from build123d import *

# Parameters (mm, degrees)
BOSS_EXTRUDE1_DEPTH          = 12.7
FILLET1_R                    = 19.05
F_10_0_1935_DIAMETER_HOLE1_D = 4.9149


with BuildPart() as part:
    # Sketch1 → Boss-Extrude1 (new body)
    with BuildSketch(Plane.ZY.offset(152.399999331)):
        Polygon((179.525, -30.525), (179.525, 10.75), (116.025, 179.025), (116.025, 191.725), (-116.025, 191.725), (-116.025, 179.025), (-179.525, 10.75), (-179.525, -30.525), align=None)
    extrude(amount=BOSS_EXTRUDE1_DEPTH)

    # Fillet1
    fillet1_edges = [part.edges().sort_by_distance(p)[0] for p in [
        (-158.749999331, 179.025, -116.025),
        (-158.749999331, 179.025, 116.025),
    ]]
    fillet(fillet1_edges, radius=FILLET1_R)

    # #10 (0.1935) Diameter Hole1 (through all)
    with Locations(Plane.ZY.offset(165.099999331)):
        with Locations((-103.325, 185.375), (-34.441666667, 185.375), (34.441666667, 185.375), (103.325, 185.375), (174.7625, -5.125), (-174.7625, -5.125), (-166.825, -25.7625), (166.825, -25.7625), (0, -25.7625), (83.4125, -25.7625), (-83.4125, -25.7625)):
            Hole(F_10_0_1935_DIAMETER_HOLE1_D / 2)


solid = part.part
Geometry: final body of the model. Coordinates: model frame, mm. A direction names the side the tool comes from. Give positions to 0.01 mm unless a question says otherwise; leave off trailing zeros. Loops run counter-clockwise (first coordinate to the right, second up) from the corner with the lowest first, then second, coordinate; pieces in that order, holes last. Notation, with made-up numbers: M -14,73 L 44,73 A21 ccw 44,105 Z; hole C 69,74 d2. An arc over 180 degrees is marked long. Put each result on its own line as item: value.
1) Material intervals for L1, parallel to Y at x = -160.5, z = 34 (3 decimals); L2, parallel to Y at x = -158, z = 0 (3 decimals); L3, parallel to Z at x = -156, y = 38, sorted ascending. Write a range as from..to.
Computed values:
L1: y = -30.525..182.958, 187.792..191.725
L2: y = -30.525..-28.22, -23.305..191.725
L3: z = -169.24..169.24
2) Reachability of faces 1 (the flat face through (-159, 187, 116.025)), 2 (the flat face through (-159, 187, -116.025)), 3 (the flat face through (-152.4, 82, -3)) from +Z, -Z, +X, -X, +Y, -Y: full face, straight path, thin tool, end or side. Return the list, or none.
Computed values:
face 1: +Z, +X, -X, +Y
face 2: -Z, +X, -X, +Y
face 3: +Z, -Z, +X, +Y, -Y
3) First-contact query: P1, Ø2, axis at x = -162.5, y = 124, coming from the -Z side; P2, Ø7.5, axis at x = -161, y = 185.5, coming from the -Z side. Flat tips, straight axial feed; report the tip coordinate or a pass-through.
Computed values:
P1: stops at z = -137.17
P2: stops at z = -116.04
4) Cut plane A-A, the plane x = -159.75. Give the number of separate pieces and of enclosed holes in the cut face, plus the area to 3 significant figures.
Computed values:
separate pieces: 1
enclosed holes: 11
area: 67,300 mm^2
5) Cut plane C-C, the plane y = 147. Return the cut outline in (x, z), plus the area to 3 significant figures.
Computed values:
outline: M -165.1,-128.11 L -152.4,-128.11 L -152.4,128.11 L -165.1,128.11 Z
area: 3,250 mm^2
6) Cut plane B-B, the plane z = -122. Return the cut outline in (x, y) (3 decimals).
Computed values:
outline: M -165.1,-30.525 L -152.4,-30.525 L -152.4,163.191 L -165.1,163.191 Z
